Read the model definition and answer for the solid it produces. Units are mm, in the model's axes. Face numbers are marked on the shaded views. A direction names the side the tool comes from. Coordinates: 2 decimals unless noted, no trailing zeros. Order: outer loops, then holes, each group sorted by start corner. A loop starts at its lowest first (then second) coordinate and runs counter-clockwise, first axis right, second up. Notation, with made-up numbers: (49.5, 82) -> (57.5, 82) arc R27 ccw to (57.5, 104) -> close; hole circle Ø5 at (-17, 31). An arc over 180 degrees is marked (long way). Use CSV: the item, a comma, the result in double quotes.
```python
from build123d import *

# Parameters (mm, degrees)
SKETCH1_W           = 40
SKETCH1_H           = 40
BOSS_EXTRUDE1_DEPTH = 12
SKETCH2_R           = 11
CUT_EXTRUDE1_DEPTH  = 7
SKETCH3_R           = 7.5
CUT_EXTRUDE2_DEPTH  = 31.724582991
FILLET1_R           = 4
SKETCH4_R           = 1.5
CUT_EXTRUDE3_DEPTH  = 31.724582991
SKETCH5_R           = 3
CUT_EXTRUDE4_DEPTH  = 3


with BuildPart() as part:
    # Sketch1 → Boss-Extrude1 (new body)
    with BuildSketch(Plane(origin=(0, 0, 0), x_dir=(1, 0, 0), z_dir=(0, 1, 0))):
        Rectangle(SKETCH1_W, SKETCH1_H)
    extrude(amount=BOSS_EXTRUDE1_DEPTH)

    # Sketch2 → Cut-Extrude1 (cut)
    with BuildSketch(Plane.XZ):
        with Locations(Location((0, 0, 0), (0, 0, 270))):
            Circle(SKETCH2_R)
    extrude(amount=-CUT_EXTRUDE1_DEPTH, mode=Mode.SUBTRACT)

    # Sketch3 → Cut-Extrude2 (cut, through all)
    with BuildSketch(Plane(origin=(0, 12, 0), x_dir=(1, 0, 0), z_dir=(0, 1, 0))):
        with Locations(Location((0, 0, 0), (0, 0, 270))):
            Circle(SKETCH3_R)
    extrude(amount=-CUT_EXTRUDE2_DEPTH, mode=Mode.SUBTRACT)

    # Fillet1
    fillet1_edges = [part.edges().sort_by_distance(p)[0] for p in [
        (20, 6, 20),
        (-20, 6, 20),
        (-20, 6, -20),
        (20, 6, -20),
    ]]
    fillet(fillet1_edges, radius=FILLET1_R)

    # Sketch4 → Cut-Extrude3 (cut, through all)
    with BuildSketch(Plane(origin=(0, 12, 0), x_dir=(1, 0, 0), z_dir=(0, 1, 0))):
        with Locations(Location((-15, 15, 0), (0, 0, 270))):
            Circle(SKETCH4_R)
        with Locations(Location((15, 15, 0), (0, 0, 90))):
            Circle(SKETCH4_R)
        with Locations(Location((15, -15, 0), (0, 0, 270))):
            Circle(SKETCH4_R)
        with Locations(Location((-15, -15, 0), (0, 0, 90))):
            Circle(SKETCH4_R)
    extrude(amount=-CUT_EXTRUDE3_DEPTH, mode=Mode.SUBTRACT)

    # Sketch5 → Cut-Extrude4 (cut)
    with BuildSketch(Plane(origin=(0, 12, 0), x_dir=(1, 0, 0), z_dir=(0, 1, 0))):
        with Locations(Location((-15, -15, 0), (0, 0, 270))):
            Circle(SKETCH5_R)
        with Locations(Location((-15, 15, 0), (0, 0, 90))):
            Circle(SKETCH5_R)
        with Locations(Location((15, -15, 0), (0, 0, 90))):
            Circle(SKETCH5_R)
        with Locations(Location((15, 15, 0), (0, 0, 270))):
            Circle(SKETCH5_R)
    extrude(amount=-CUT_EXTRUDE4_DEPTH, mode=Mode.SUBTRACT)


solid = part.part
```
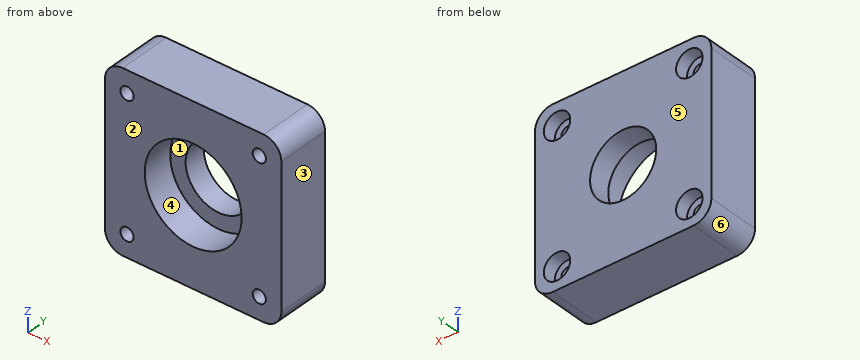
Item 1: Find section D-D, the plane x = 15. Give the vertices of the cut face in (y, z).
Return value:
outline,"(0, -20) -> (12, -20) -> (12, -18) -> (9, -18) -> (9, -16.5) -> (0, -16.5) -> close; (0, -13.5) -> (9, -13.5) -> (9, -12) -> (12, -12) -> (12, 12) -> (9, 12) -> (9, 13.5) -> (0, 13.5) -> close; (0, 16.5) -> (9, 16.5) -> (9, 18) -> (12, 18) -> (12, 20) -> (0, 20) -> close"
Item 2: Each of these flat-tipped pins is pushed along its axis until it touches: P1, Ø5, axis at x = 4.5, z = 10, coming from the -Y side; P2, Ø3.5, axis at x = -15, z = 15, coming from the +Y side. Where does it stop, or does it pass through?
Return value:
P1,"stops at y = 0"
P2,"stops at y = 9"
Item 3: The mould has two halves that part along X. Classify the marked faces 3, 4, 5 and 6: +X half, -X half, draft (parallel to the pull), parting line (faces both ways), or undercut.
Return value:
face 3,"+X half"
face 4,"undercut"
face 5,"draft"
face 6,"-X half"
Item 4: Find section C-C, the plane y = 11. Give the vertices of the cut face in (x, z), then the cut area to 3 significant figures.
Return value:
outline,"(-20, -16) arc R4 ccw to (-16, -20) -> (16, -20) arc R4 ccw to (20, -16) -> (20, 16) arc R4 ccw to (16, 20) -> (-16, 20) arc R4 ccw to (-20, 16) -> close; hole circle Ø6 at (-15, -15); hole circle Ø6 at (-15, 15); hole circle Ø15 at (0, 0); hole circle Ø6 at (15, -15); hole circle Ø6 at (15, 15)"
area,"1,300 mm^2"
Item 5: Straight lines are drawn through the part: line 1 along X through (y, z) = (5, 15); line 2 along X through (y, z) = (4.5, 0); line 3 along Z through (x, y) = (14.5, 1.75). For each, find the intervals that lie inside material, in ascending order.
Return value:
line 1,"x = -20 to -16.5, -13.5 to 13.5, 16.5 to 20"
line 2,"x = -20 to -11, 11 to 20"
line 3,"z = -20 to -16.41, -13.59 to 13.59, 16.41 to 20"
Item 6: A tool of negligible diameter and unlimited length cuts with its end or side. For the marked faces 1 and 2, from which of +Z, -Z, +X, -X, +Y, -Y can it reach the whole face along a straight path? Write none if from no direction.
Return value:
face 1,"-Y"
face 2,"+Z, -Z, +X, -X, -Y"
Item 7: Find section A-A, the plane x = 0. Give the vertices of the cut face in (y, z), then the cut area to 3 significant figures.
Return value:
outline,"(0, -20) -> (12, -20) -> (12, -7.5) -> (7, -7.5) -> (7, -11) -> (0, -11) -> close; (0, 11) -> (7, 11) -> (7, 7.5) -> (12, 7.5) -> (12, 20) -> (0, 20) -> close"
area,"251 mm^2"
Item 8: Find section B-B, the plane z = -15. Give the vertices of the cut face in (x, y), then the cut area to 3 significant figures.
Return value:
outline,"(-20, 0) -> (-16.5, 0) -> (-16.5, 9) -> (-18, 9) -> (-18, 12) -> (-20, 12) -> close; (-13.5, 0) -> (13.5, 0) -> (13.5, 9) -> (12, 9) -> (12, 12) -> (-12, 12) -> (-12, 9) -> (-13.5, 9) -> close; (16.5, 0) -> (20, 0) -> (20, 12) -> (18, 12) -> (18, 9) -> (16.5, 9) -> close"
area,"390 mm^2"
